```python
from build123d import *

# Parameters (mm, degrees)
F0_W     = 35
F0_H     = 20
F1_DEPTH = 12
F2_T     = -1.8
F3_DEPTH = 2


with BuildPart() as f1:
    # F0 (on Top) → F1 (new body)
    with BuildSketch(Plane.XY):
        Polygon((-19.0813283622, 35.3948845826), (-34.0813283622, 35.3948845826), (-34.0813283622, -14.6051154174), (-19.0813283622, -14.6051154174), (-19.0813283622, 5.3948845826), align=None)
        with Locations((-1.5813283622, -4.6051154174)):
            Rectangle(F0_W, F0_H)
    extrude(amount=F1_DEPTH)

    # F2
    f2_openings = [f1.faces().sort_by_distance(p)[0] for p in [
        (-14.512363, 3.153505, 12),
    ]]
    offset(amount=F2_T, openings=f2_openings, kind=Kind.INTERSECTION)

    # F0 (on Top) → F3 (cut)
    with BuildSketch(Plane.XY):
        Polygon((-19.0813283622, 35.3948845826), (-34.0813283622, 35.3948845826), (-34.0813283622, -14.6051154174), (-19.0813283622, -14.6051154174), (-19.0813283622, 5.3948845826), align=None)
        with Locations((-1.5813283622, -4.6051154174)):
            Rectangle(F0_W, F0_H)
    extrude(amount=F3_DEPTH, mode=Mode.SUBTRACT)


solid = f1.part
```
CAD build for the part. Positions are in the model's coordinates, mm. A direction names the side the tool comes from. Round coordinates to 2 decimals unless told otherwise and drop trailing zeros. Order: outer loops, then holes, each group sorted by start corner. A loop starts at its lowest first (then second) coordinate and runs counter-clockwise, first axis right, second up.
Item 1: Pin check, flat tips, straight feed: pin 1 (5 mm diameter, centred on y = 22, z = 10.5, fed in from +X); pin 2 (3 mm diameter, centred on x = -12, z = 5, fed in from +Y). Stop position of each tip, or through.
Item 2: Probe line 1 along X through (y, z) = (19, 10.25); line 2 along Y through (x, z) = (-9, 10.75); line 3 along X through (y, z) = (-4, 6.5). List the from-to ranges inside material, lowest first.
Item 3: Saw through at B-B on y = 11. Write the cut outline in (x, z).
Item 4: Mould opens along Y. For faces 1 (the face through (-19.081, 20, 7)), 2 (the face through (14.119, -5, 7)), 3 (the face through (-9, -14.605, 7)), 4 (the face through (-26, 35.395, 7)) say: pulls with the +Y half, pulls with the -Y half, needs draft (parallel to the pull), parting line crosses it, or undercut.
Item 5: Tool access for faces 5 (the face through (-34.081, 11, 7)), 6 (the face through (-32.281, 11, 7)), 7 (the face through (-2, 5.395, 7)): list every direction of +Z, -Z, +X, -X, +Y, -Y with a clear straight run to the whole face (end or side of a thin tool).
Item 6: Saw through at A-A on x = 8. Write the cut outline in (y, z).
Item 7: Saw through at C-C on z = 6.5. Write the cut outline in (x, y), then the cut area to 3 significant figures.
Reported:
1. pin 1: stops at x = -19.08
1. pin 2: stops at y = 5.39
2. line 1: x = -34.08 to -32.28, -20.88 to -19.08
2. line 2: y = -14.61 to -12.81, 3.59 to 5.39
2. line 3: x = -34.08 to -32.28, 14.12 to 15.92
3. outline: (-34.08, 2) - (-32.28, 2) - (-32.28, 12) - (-34.08, 12) - close; (-20.88, 2) - (-19.08, 2) - (-19.08, 12) - (-20.88, 12) - close
4. face 1: needs draft
4. face 2: undercut
4. face 3: pulls with the -Y half
4. face 4: pulls with the +Y half
5. face 5: +Z, -Z, -X, +Y, -Y
5. face 6: +Z, -Z
5. face 7: +Z, -Z, +X, +Y
6. outline: (-14.61, 2) - (-12.81, 2) - (-12.81, 12) - (-14.61, 12) - close; (3.59, 2) - (5.39, 2) - (5.39, 12) - (3.59, 12) - close
7. outline: (-34.08, -14.61) - (15.92, -14.61) - (15.92, 5.39) - (-19.08, 5.39) - (-19.08, 35.39) - (-34.08, 35.39) - close; hole (-32.28, -12.81) - (14.12, -12.81) - (14.12, 3.59) - (-20.88, 3.59) - (-20.88, 33.59) - (-32.28, 33.59) - close
7. area: 347 mm2
